Input: dimensioned drawing with shaded views. Units: mm. Origin: part minimum x, y, z. Round coordinates to 2 decimals unless told otherwise and drop trailing zeros. Write each loop counter-clockwise with the first axis right and the second up, starting at its lowest first coordinate (ties: lowest second). Pieces come first, ordered by that corner, then holes. Notation, with made-up numbers: M 70.5,66.5 L 106.5,66.5 A28 cw 106.5,104.5 Z; hole C 30.25,32.25 d2. An arc over 180 degrees is marked long. Use one line per item in the form item = value. Start each with the question number.
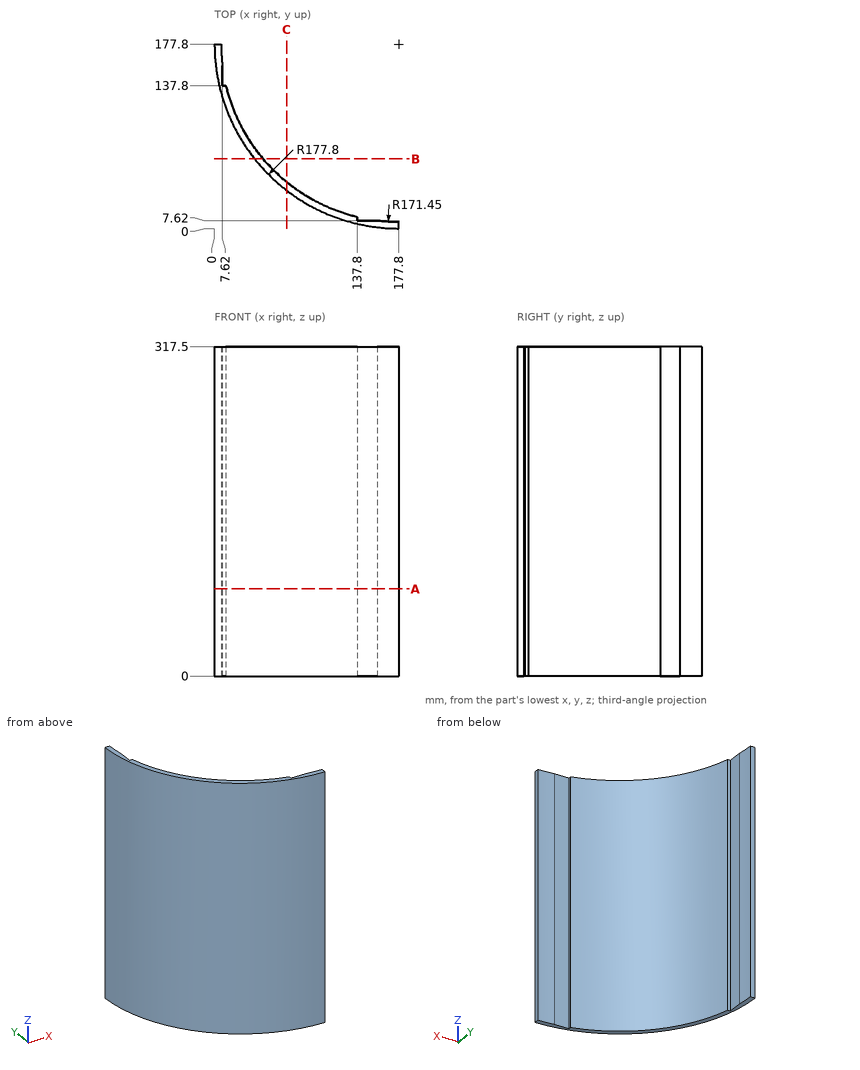
1. Section query B-B (y = 67). Return loops of the section in (x, z), then the cut area to 3 significant figures.
2. Ray query, probe 1 along X at (y, z) = (158, 31); probe 2 along X at (y, z) = (121, 134.5); probe 3 along Y at (x, z) = (165.5, 231). Return the intervals inside material, ascending.
3. Section query A-A (z = 84). Return loops of the section in (x, y).
4. Section query C-C (x = 69.5). Return loops of the section in (y, z).
5. Contact query for flat-ended pins moving along their axis: pin 1 (1 mm diameter, centred on x = 9.5, z = 201.5, fed in from +Y); pin 2 (6 mm diameter, centred on x = 146.5, z = 92.5, fed in from +Y); pin 3 (8 mm diameter, centred on x = 129.5, z = 189, fed in from +Y). Output: stop coordinate, or through.
Checks:
q1.outline = M 38.75,0 L 46.96,0 L 46.96,317.5 L 38.75,317.5 Z
q1.area = 2,610 mm^2
q2.probe_1 = 1.11 to 7.5
q2.probe_2 = 9.32 to 16.03
q2.probe_3 = 0.43 to 6.79
q3.outline = M 0,177.8 A177.8 ccw 177.8,0 L 177.8,6.35 A171.45 cw 156.97,7.62 L 137.8,7.62 L 137.8,11.08 A171.45 cw 11.08,137.8 L 7.62,137.8 L 7.62,156.97 A171.45 cw 6.35,177.8 Z
q4.outline = M 36.79,0 L 44.89,0 L 44.89,317.5 L 36.79,317.5 Z
q5.pin_1 = 137.8
q5.pin_2 = 7.62
q5.pin_3 = 14.52
